Autodesk Inventor part; units mm, degrees
ref_plane "YZ Plane" through (0, 0, 0) normal (1, 0, 0) x (0, 1, 0)
ref_plane "XZ Plane" through (0, 0, 0) normal (0, 1, 0) x (-1, 0, 0)
ref_plane "XY Plane" through (0, 0, 0) normal (0, 0, 1) x (1, 0, 0)
sketch "Sketch1" plane through (0, 0, 0) normal (0, 1, 0) x (-1, 0, 0)
  line L0 (0, 0) -> (120, 0)
  line L1 (120, 0) -> (120, -150.5)
  line L2 (120, -150.5) -> (0, -150.5)
  line L3 (0, -150.5) -> (0, 0)
  line L4 (118, -148.5) -> (118, -2)
  line L5 (118, -2) -> (2, -2)
  line L6 (0, -148.5) -> (118, -148.5)
  line L7 (2, -2) -> (0, -2)
  line L8 (1.5, -2) -> (1.5, -148.5)
  point P0 (0, -144.5)
  dimension "d0" = 150.5
  dimension "d1" = 120
  dimension "d2" = 2
  dimension "d3" = 1.5
  dimension "d13" = 2
  dimension "d14" = 2
extrude "Extrusion1" add sketch "Sketch1" along normal blind 52 contours L0 L1 L2 L3 L6 L4 L5 L7
sketch "Sketch2" plane through (0, 0, 0) normal (0, -1, 0) x (1, 0, 0)
  line L0 (-120, -150.5) -> (-120, 0)
  line L1 (0, -150.5) -> (-120, -150.5)
  line L2 (0, -148.5) -> (0, -150.5)
  line L3 (-118, -148.5) -> (0, -148.5)
  line L4 (0, 0) -> (0, -2)
  line L5 (-120, 0) -> (0, 0)
  line L6 (0, -150.5) -> (-120, -150.5)
  line L7 (-120, -150.5) -> (-120, 0)
  line L8 (-120, 0) -> (0, 0)
  line L9 (0, 0) -> (0, -150.5)
  line L10 (-118, -2) -> (-118, -148.5)
  line L11 (0, -2) -> (-118, -2)
extrude "Extrusion2" add sketch "Sketch2" along normal blind 2
sketch "Sketch3" plane through (0, 0, 0) normal (0, 1, 0) x (1, 0, 0)
  line L0 (0, 2) -> (-118, 2)
  line L1 (0, 148.5) -> (0, 2)
  line L2 (-118, 148.5) -> (0, 148.5)
  line L3 (-118, 2) -> (-118, 148.5)
  line L4 (-3.2, 2) -> (-3.2, 148.5)
  circle A0 centre (-118, 2) radius 2
  line L5 (-120, 0) -> (-120, 150.5)
  circle A1 centre (-118, 148.5) radius 2
  circle A2 centre (-5.2, 2) radius 2
  line L6 (-120, 0) -> (0, 0)
  line L7 (-5.2, 4) -> (-3.2, 4)
  circle A3 centre (-5.2, 148.5) radius 2
  line L8 (-5.2, 146.5) -> (-3.2, 146.5)
  circle A4 centre (-118, 75.25) radius 2
  line L9 (0, 150.5) -> (-120, 150.5)
  circle A5 centre (-37.2167, 2) radius 2
  circle A6 centre (-37.2167, 148.5) radius 2
  point P0 (-59, 2)
  point P1 (-7.2, 148.5)
  point P2 (-3.2, 146.5)
  point P3 (-3.2, 148.5)
  point P4 (-7.2, 2)
  point P5 (-118, 146.5)
  point P6 (-116, 148.5)
  point P7 (-116, 2)
  point P8 (-118, 4)
  point P9 (-118, 73.25)
  point P10 (-118, 77.25)
  dimension "d15" = 3.2
extrude "Extrusion3" add sketch "Sketch3" along normal up to surface (52 mm away) contours A2 L0 | A2 L7 L4 | L0 A2 | A3 L2 | L4 L8 A3 | L2 A3 | A5 L0 | L0 A5 | A0 L3 L0 | A6 L2 | L2 A6 | L0 L3 A0 | A1 L2 L3 | A4 L3 | A1 L3 L2 | L3 A4
sketch "Sketch6" plane through (0, 0, -2) normal (0, 0, -1) x (-1, 0, 0)
  line L0 (5.2, 52) -> (3.2, 52)
  line L1 (3.2, 0) -> (3.2, 52)
  line L2 (5.2, 0) -> (3.2, 0)
  line L3 (5.2, 0) -> (5.2, 52)
  line L4 (7.2, 52) -> (7.2, 0)
  line L5 (7.2, 52) -> (5.2, 52)
  line L6 (5.2, 0) -> (5.2, 52)
  line L7 (7.2, 0) -> (5.2, 0)
  line L8 (3.2, 0) -> (5.2, 0)
  line L9 (5.2, 0) -> (5.2, 3.2)
  line L10 (5.2, 3.2) -> (3.2, 3.2)
  line L11 (3.2, 3.2) -> (3.2, 0)
  arc A0 (7.2, 0) -> (5.2, 3.2) centre (3.64, 0) ccw
  point P0 (0, 0)
  point P1 (3.2, 3.2)
  dimension "d29" = 3.2
extrude "Extrusion5" add sketch "Sketch6" along normal through all contours A0 L7 L3 | L3 L2 L1 L10
sketch "Sketch7" plane through (0, 0, 0) normal (0, 1, 0) x (1, 0, 0)
  line L0 (-7.2, 2) -> (-3.2, 2)
  line L1 (-3.2, 4) -> (-3.2, 146.5)
  circle A0 centre (-73.7868, 6.5) radius 1.5
  circle A1 centre (-73.7868, 36) radius 1.5
  line L2 (-39.2167, 2) -> (-116, 2)
  line L3 (-77.4105, 0.6903) -> (-77.4105, 39.7313) construction
  line L4 (-77.4105, 39.7313) -> (-39.4979, 39.7313) construction
  line L5 (-39.4979, 39.7313) -> (-39.4979, 0.6903) construction
  line L6 (-39.4979, 0.6903) -> (-77.4105, 0.6903) construction
  circle A2 centre (-43.2868, 23.5) radius 1.5
  circle A3 centre (-73.7868, 6.5) radius 2.75
  circle A4 centre (-73.7868, 36) radius 2.75
  circle A5 centre (-43.2868, 23.5) radius 2.75
  point P0 (0, 0)
  point P1 (-57, 2)
  dimension "d35" = 29.5
  dimension "d38" = 3
  dimension "d39" = 3
  dimension "d40" = 4.5
  dimension "d68" = 3
  dimension "d69" = 30.5
  dimension "d70" = 12.5
  dimension "d71" = 5.5
  dimension "d72" = 5.5
  dimension "d73" = 5.5
extrude "Extrusion6" add sketch "Sketch7" along normal blind 6 contours A0 | A1 | A2 | A3 | A4 | A5
sketch "Sketch8" plane through (0, 0, 0) normal (0, 1, 0) x (1, 0, 0)
  circle A0 centre (-49.2001, 130.9565) radius 3
  circle A1 centre (-49.2001, 59.7565) radius 3
  circle A2 centre (-95.4, 59.7565) radius 3
  circle A3 centre (-95.4, 130.9565) radius 3
  circle A4 centre (-49.2001, 130.9565) radius 3
  circle A5 centre (-49.2001, 59.7565) radius 3
  circle A6 centre (-95.4, 59.7565) radius 3
  circle A7 centre (-95.4, 130.9565) radius 3
  point P0 (0, 0)
  point P1 (-129.8781, 142.9288)
  dimension "d76" = 71.2
  dimension "d77" = 46.2
extrude "Extrusion7" add sketch "Sketch8" along normal blind 6
equation "\"d13\" = d2"
properties part number "controller-base"
The model under review builds one solid part; all positions refer to its coordinate system, in mm. A direction names the side the tool comes from. Give positions to 0.01 mm unless a question says otherwise; leave off trailing zeros. Write each loop counter-clockwise with the first axis right and the second up, starting at its lowest first coordinate (ties: lowest second). Pieces come first, ordered by that corner, then holes.
1. Add section B-B, the plane y = 33. Write out the cut boundary in (x, z), plus the area to 3 significant figures.
2. Draft analysis for pull direction X (two halves, no side actions). For faces 1 (the cylindrical face through (-37.3, 25.6, -4)), 2 (the flat face through (-120, 25, -74)), 3 (the flat face through (-2, 26, -148.5)), state which applies: +X half, -X half, draft (parallel to the pull), parting line (faces both ways), or undercut.
3. Wall thickness on L1, parallel to Z at x = -40, y = 6; L2, parallel to Y at x = -86, z = -126; L3, parallel to X at y = 11, z = -101.5: over which ranges is each line inside the solid? List them lowest first.
4. Add section D-D, the plane x = -95.4. Write out the cut boundary in (y, z), plus the area to 3 significant figures.
5. Tool access review of faces 4 (the flat face through (-59, 25, 0)), 5 (the flat face through (-21, 26, -148.5)), 6 (the flat face through (-95, 6, -60)): name each direction out of +Z, -Z, +X, -X, +Y, -Y from which nothing blocks a thin tool from reaching the whole face with its end or side.
6. For P1, Ø3, axis at x = -95, z = -61, coming from the +Y side; P2, Ø1, axis at x = -4.5, z = -101, coming from the +Y side; P3, Ø1.6, axis at x = -4.5, y = 19, coming from the +Z side; P4, Ø2, axis at y = 43.5, z = -19, coming from the +X side, all flat-tipped, find the tip position at first contact; note any pin that passes through.
7. Add section C-C, the plane z = -23.5. Write out the cut boundary in (x, y), plus the area to 3 significant figures.
8. Add section A-A, the plane x = -67. Write out the cut boundary in (y, z).
Worked answers:
1. outline: (-120, -150.5) - (0, -150.5) - (0, -148.5) - (-3.2, -148.5) - (-3.2, -146.5) - (-5.2, -146.5) arc R2 ccw to (-7.2, -148.5) - (-35.22, -148.5) arc R2 ccw to (-39.22, -148.5) - (-116, -148.5) arc R2 ccw to (-118, -146.5) - (-118, -77.25) arc R2 ccw to (-118, -73.25) - (-118, -4) arc R2 ccw to (-116, -2) - (-39.22, -2) arc R2 ccw to (-35.22, -2) - (-7.2, -2) arc R2 ccw to (-5.2, -4) - (-3.2, -4) - (-3.2, -2) - (0, -2) - (0, 0) - (-120, 0) - close
1. area: 812 mm2
2. face 1: undercut
2. face 2: -X half
2. face 3: draft
3. L1: z = -150.5 to -148.5, -2 to 0
3. L2: y = -2 to 0
3. L3: x = -120 to -118
4. outline: (-2, -150.5) - (52, -150.5) - (52, -148.5) - (0, -148.5) - (0, -133.96) - (6, -133.96) - (6, -127.96) - (0, -127.96) - (0, -62.76) - (6, -62.76) - (6, -56.76) - (0, -56.76) - (0, -2) - (52, -2) - (52, 0) - (-2, 0) - close
4. area: 581 mm2
5. face 4: +Z, +X, -X, +Y, -Y
5. face 5: +Y
5. face 6: +X, +Y
6. P1: stops at y = 6
6. P2: stops at y = 3.2
6. P3: stops at z = 0
6. P4: stops at x = -118
7. outline: (-120, -2) - (0, -2) - (0, 0) - (-3.2, 0) - (-3.2, 3.2) - (-5.2, 3.2) arc R3.56 ccw to (-7.2, 0) - (-40.54, 0) - (-40.54, 6) - (-46.04, 6) - (-46.04, 0) - (-118, 0) - (-118, 52) - (-120, 52) - close
7. area: 388 mm2
8. outline: (-2, -150.5) - (52, -150.5) - (52, -148.5) - (0, -148.5) - (0, -2) - (52, -2) - (52, 0) - (-2, 0) - close
